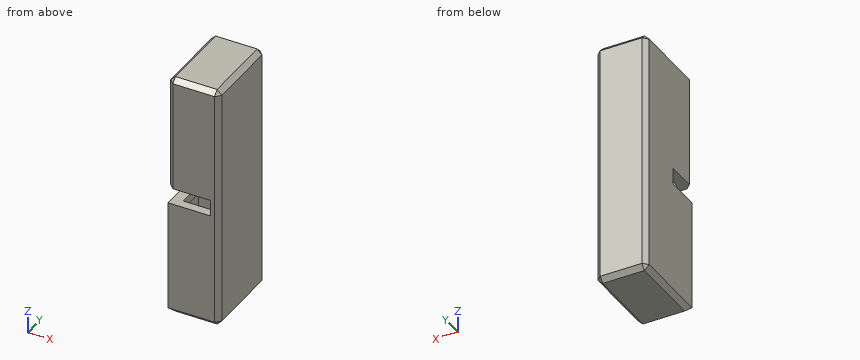
```python
from build123d import *

# Parameters (mm, degrees)
SKETCH1_W                       = 75
SKETCH1_H                       = 120
BOSS_EXTRUDE1_DEPTH             = 181.5
SKETCH2_W                       = 24
SKETCH2_H                       = 50
CUT_EXTRUDE1_DEPTH              = 15
SHELL1_START                    = -22.5
SHELL1_OUTLINE_W                = 94
SHELL1_OUTLINE_H                = 337
SHELL1_DEPTH                    = 47
SHELL1_START_2                  = -24.5
SHELL1_2_DEPTH                  = 2
BOSS_EXTRUDE2_REACH             = 196.804
SKETCH3_W                       = 45
SKETCH3_H                       = 13
BOSS_EXTRUDE2_DIRECTION_2_REACH = 196.804
CHAMFER1_SIZE                   = 7
CUT_EXTRUDE2_START              = -62
SKETCH4_W                       = 24
SKETCH4_H                       = 104.028076608
CUT_EXTRUDE2_DEPTH              = 49


# Read off the part's stored shape, not the designer's step: Shell1
with BuildPart() as part:
    # Sketch1 → Boss-Extrude1 (new, symmetric)
    with BuildSketch(Plane.XY):
        Rectangle(SKETCH1_W, SKETCH1_H)
    extrude(amount=BOSS_EXTRUDE1_DEPTH, both=True)

    # Sketch2 → Cut-Extrude1 (cut)
    with BuildSketch(Plane(origin=(-37.5, 0, 131.5), x_dir=(0, 0, -1), z_dir=(1, 0, 0))):
        with Locations((131.5, -35)):
            Rectangle(SKETCH2_W, SKETCH2_H)
    extrude(amount=CUT_EXTRUDE1_DEPTH, mode=Mode.SUBTRACT)

    # Shell1 outline → Shell1 (cut)
    with BuildSketch(Plane.YZ.offset(SHELL1_START)):
        Rectangle(SHELL1_OUTLINE_W, SHELL1_OUTLINE_H)
    extrude(amount=SHELL1_DEPTH, mode=Mode.SUBTRACT)

    # Shell1 2 outline → Shell1 2 (cut)
    with BuildSketch(Plane.YZ.offset(SHELL1_START_2)):
        Polygon((-47, -25), (-47, -168.5), (47, -168.5), (47, 168.5), (-47, 168.5), (-47, 25), (3, 25), (3, -25), align=None)
    extrude(amount=SHELL1_2_DEPTH, mode=Mode.SUBTRACT)

    # Sketch3 → Boss-Extrude2 (add, up to next)
    with BuildSketch(Plane.XY, mode=Mode.PRIVATE) as boss_extrude2_sk1:
        Rectangle(SKETCH3_W, SKETCH3_H)
    boss_extrude2_tool1 = extrude(boss_extrude2_sk1.sketch, amount=-BOSS_EXTRUDE2_REACH, mode=Mode.PRIVATE) - part.part
    add(boss_extrude2_tool1.solids().sort_by_distance((0, 0, 0))[0])

    # Sketch3 → Boss-Extrude2 direction 2 (add, up to next)
    with BuildSketch(Plane.XY, mode=Mode.PRIVATE) as boss_extrude2_direction_2_sk1:
        Rectangle(SKETCH3_W, SKETCH3_H)
    boss_extrude2_direction_2_tool1 = extrude(boss_extrude2_direction_2_sk1.sketch, amount=BOSS_EXTRUDE2_DIRECTION_2_REACH, mode=Mode.PRIVATE) - part.part
    add(boss_extrude2_direction_2_tool1.solids().sort_by_distance((0, 0, 0))[0])

    # Chamfer1
    chamfer1_edges = [part.edges().sort_by_distance(p)[0] for p in [
        (0, -60, 181.5),
        (37.5, 0, 181.5),
        (0, 60, 181.5),
        (37.5, 0, -181.5),
        (0, -60, -181.5),
        (-37.5, 0, -181.5),
        (0, 60, -181.5),
        (-37.5, 0, 181.5),
        (37.5, 60, 0),
        (37.5, -60, 0),
        (-37.5, -60, 96.75),
        (-37.5, 60, 0),
    ]]
    chamfer(chamfer1_edges, length=CHAMFER1_SIZE)

    # Sketch4 → Cut-Extrude2 (cut)
    with BuildSketch(Plane.ZY.offset(37.5).offset(CUT_EXTRUDE2_START)):
        with Locations((0, -20.489530189)):
            Rectangle(SKETCH4_W, SKETCH4_H)
    extrude(amount=CUT_EXTRUDE2_DEPTH, mode=Mode.SUBTRACT)


solid = part.part
```
CAD build for the part. Positions are in the model's coordinates, mm. Round coordinates to 2 decimals unless told otherwise and drop trailing zeros. Order: outer loops, then holes, each group sorted by start corner. A loop starts at its lowest first (then second) coordinate and runs counter-clockwise, first axis right, second up. Notation, with made-up numbers: (34, 78) -> (62, 78) arc R24 ccw to (62, 111) -> close; hole circle Ø2 at (29, -5). An arc over 180 degrees is marked (long way). One line per question, with ' | ' between items.
Q1. Slice it at A-A (z = 136.5). Write the cut outline in (x, y), then the cut area to 3 significant figures.
Completed:
outline: (-37.5, -53) -> (-30.5, -60) -> (30.5, -60) -> (37.5, -53) -> (37.5, 53) -> (30.5, 60) -> (-30.5, 60) -> (-37.5, 53) -> close; (-22.5, -6.5) -> (22.5, -6.5) -> (22.5, 6.5) -> (-22.5, 6.5) -> close; hole (-24.5, -47) -> (24.5, -47) -> (24.5, 47) -> (-24.5, 47) -> close | area: 4,880 mm^2
Q2. Probe probe 1 along Y at (x, z) = (21.5, -66.5); probe 2 along X at (y, z) = (3, 48); probe 3 along Y at (x, z) = (-23, -44). List the from-to ranges inside material, lowest first.
Completed:
probe 1: y = -60 to -47, -6.5 to 6.5, 47 to 60 | probe 2: x = -37.5 to -24.5, -22.5 to 22.5, 24.5 to 37.5 | probe 3: y = -60 to -47, 47 to 60
Q3. Slice it at D-D (y = 22). Write the cut outline in (x, z).
Completed:
outline: (-37.5, -174.5) -> (-30.5, -181.5) -> (30.5, -181.5) -> (37.5, -174.5) -> (37.5, 174.5) -> (30.5, 181.5) -> (-30.5, 181.5) -> (-37.5, 174.5) -> close; hole (-24.5, -168.5) -> (24.5, -168.5) -> (24.5, 168.5) -> (-24.5, 168.5) -> close
Q4. Slice it at C-C (z = -3). Write the cut outline in (x, y).
Completed:
outline: (-37.5, -10) -> (-24.5, -10) -> (-24.5, 47) -> (24.5, 47) -> (24.5, -60) -> (30.5, -60) -> (37.5, -53) -> (37.5, 53) -> (30.5, 60) -> (-30.5, 60) -> (-37.5, 53) -> close
Q5. Slice it at B-B (y = -14). Write the cut outline in (x, z).
Completed:
outline: (-37.5, -174.5) -> (-30.5, -181.5) -> (30.5, -181.5) -> (37.5, -174.5) -> (37.5, 174.5) -> (30.5, 181.5) -> (-30.5, 181.5) -> (-37.5, 174.5) -> (-37.5, 12) -> (-22.5, 12) -> (-22.5, 25) -> (-24.5, 25) -> (-24.5, 168.5) -> (24.5, 168.5) -> (24.5, -168.5) -> (-24.5, -168.5) -> (-24.5, -25) -> (-22.5, -25) -> (-22.5, -12) -> (-37.5, -12) -> close
